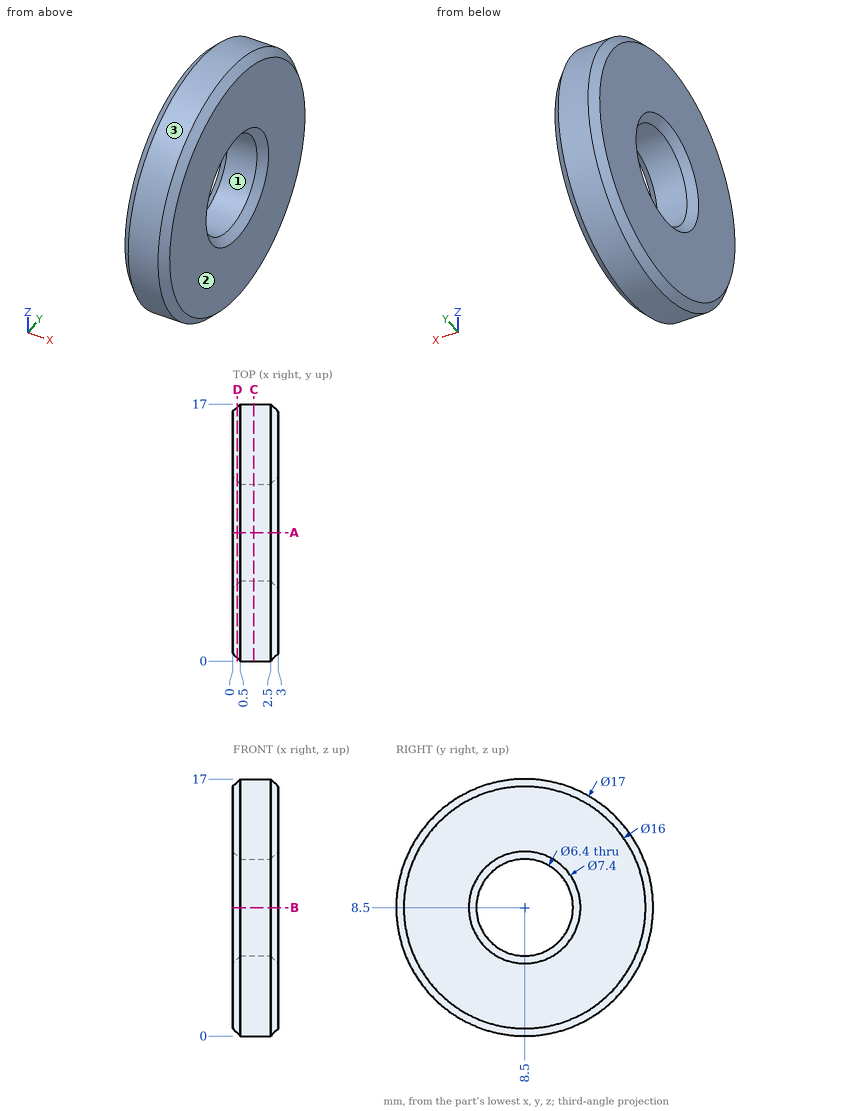
Here's the drawing with two shaded views (mm, measured from the low corner). I have some questions. Round coordinates to 2 decimals unless told otherwise and drop trailing zeros. Loops run counter-clockwise (first coordinate to the right, second up) from the corner with the lowest first, then second, coordinate; pieces in that order, holes last.
Item 1: Suppose I cut it at C-C, the plane x = 1.4. Write out the boundary of the cut face in (y, z), then the cut area to 3 significant figures.
Item 2: Will these pins go through, and if not, where does the flat tip stop? pin 1 Ø1.5 at (x, z) = (1.5, 5.5) entering from +Y; pin 2 Ø1 at (x, y) = (1, 3) entering from -Z; pin 3 Ø1 at (x, z) = (1.5, 12.5) entering from +Y.
Item 3: Suppose I cut it at A-A, the plane y = 8.5. Write out the boundary of the cut face in (x, z), then the cut area to 3 significant figures.
Item 4: If we mould it in two halves opening along Z, with no side actions, what happens to the marked faces 1, 2 and 3? For each: +Z half, -Z half, draft (parallel to the pull), parting line (faces both ways), or undercut.
Item 5: Please list where these lines run through material, in increasing order: L1, parallel to Y at x = 1.8, z = 8.5; L2, parallel to Z at x = 2, y = 11; L3, parallel to Y at x = 2.65, z = 6.5.
Item 6: Suppose I cut it at D-D, the plane x = 0.3. Write out the boundary of the cut face in (y, z), then the cut area to 3 significant figures.
Reported:
1. outline: circle Ø17 at (8.5, 8.5); hole circle Ø6.4 at (8.5, 8.5)
1. area: 195 mm2
2. pin 1: stops at y = 16.7
2. pin 2: stops at z = 1.63
2. pin 3: stops at y = 16.25
3. outline: (0, 0.5) - (0.5, 0) - (2.5, 0) - (3, 0.5) - (3, 4.8) - (2.5, 5.3) - (0.5, 5.3) - (0, 4.8) - close; (0, 12.2) - (0.5, 11.7) - (2.5, 11.7) - (3, 12.2) - (3, 16.5) - (2.5, 17) - (0.5, 17) - (0, 16.5) - close
3. area: 30.8 mm2
4. face 1: undercut
4. face 2: draft
4. face 3: parting line
5. L1: y = 0 to 5.3, 11.7 to 17
5. L2: z = 0.38 to 6.5, 10.5 to 16.62
5. L3: y = 0.39 to 5.81, 11.19 to 16.61
6. outline: circle Ø16.6 at (8.5, 8.5); hole circle Ø6.8 at (8.5, 8.5)
6. area: 180 mm2
